```python
from build123d import *

# Parameters (mm, degrees)
SKETCH1_R           = 150
BOSS_EXTRUDE1_DEPTH = 3
SKETCH2_R           = 3.5
CUT_EXTRUDE1_DEPTH  = 3
CIRPATTERN1_COUNT   = 3
SKETCH3_R           = 2
CUT_EXTRUDE2_DEPTH  = 3
SKETCH4_R           = 15
CUT_EXTRUDE3_DEPTH  = 3
SKETCH6_R           = 1.5
CUT_EXTRUDE5_DEPTH  = 3


with BuildPart() as part:
    # Sketch1 → Boss-Extrude1 (new body)
    with BuildSketch(Plane.XY):
        Circle(SKETCH1_R)
    extrude(amount=BOSS_EXTRUDE1_DEPTH)

    # Sketch2 → Cut-Extrude1 (cut)
    with BuildSketch(Plane(origin=(0, 0, 0), x_dir=(-1, 0, 0), z_dir=(0, 0, -1))):
        with Locations((-84.532410842, 88.488821425)):
            Circle(SKETCH2_R)
        with Locations(Location((-112.064079787, 49.169523299, 0), (0, 0, 180))):
            Circle(SKETCH2_R)
    cut_extrude1 = extrude(amount=-CUT_EXTRUDE1_DEPTH, mode=Mode.SUBTRACT)

    # CirPattern1: Cut-Extrude1 ×3 about axis
    cirpattern1_axis = Axis((0, 0, 0), (0, 0, 1))
    for i in range(1, CIRPATTERN1_COUNT):
        add(cut_extrude1.rotate(cirpattern1_axis, i * 360 / CIRPATTERN1_COUNT), mode=Mode.SUBTRACT)

    # Sketch3 → Cut-Extrude2 (cut)
    with BuildSketch(Plane(origin=(0, 0, 0), x_dir=(-1, 0, 0), z_dir=(0, 0, -1))):
        with Locations((-109.9539568, -12.654144936)):
            Circle(SKETCH3_R)
        with Locations((-80.370678478, -76.095690029)):
            Circle(SKETCH3_R)
    extrude(amount=-CUT_EXTRUDE2_DEPTH, mode=Mode.SUBTRACT)

    # Sketch4 → Cut-Extrude3 (cut)
    with BuildSketch(Plane(origin=(0, 0, 0), x_dir=(-1, 0, 0), z_dir=(0, 0, -1))):
        Circle(SKETCH4_R)
    extrude(amount=-CUT_EXTRUDE3_DEPTH, mode=Mode.SUBTRACT)

    # Sketch6 → Cut-Extrude5 (cut)
    with BuildSketch(Plane(origin=(0, 0, 0), x_dir=(-1, 0, 0), z_dir=(0, 0, -1))):
        with Locations((66.962630167, -75.769427615)):
            Circle(SKETCH6_R)
        with Locations((86.113741245, -91.839117858)):
            Circle(SKETCH6_R)
        with Locations((105.397369535, -68.857784564)):
            Circle(SKETCH6_R)
        with Locations((86.246258457, -52.788094322)):
            Circle(SKETCH6_R)
    extrude(amount=-CUT_EXTRUDE5_DEPTH, mode=Mode.SUBTRACT)


solid = part.part
```
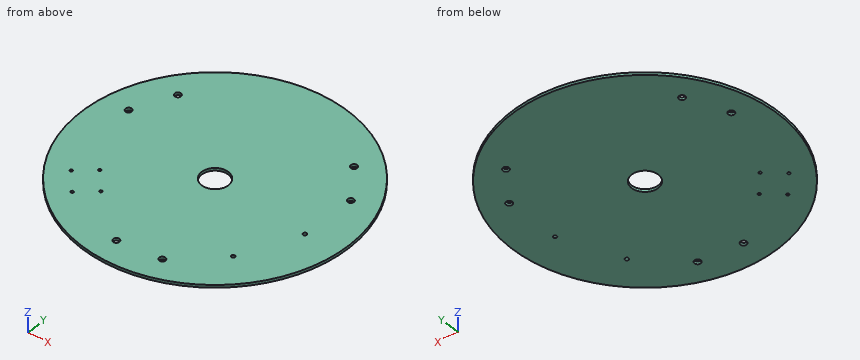
Part model, mm, in its own coordinate system. Round coordinates to 2 decimals unless told otherwise and drop trailing zeros. Loops run counter-clockwise (first coordinate to the right, second up) from the corner with the lowest first, then second, coordinate; pieces in that order, holes last.
1. Flat gauge pins, fed straight in: pin 1 (1 mm diameter, centred on x = -34, y = -31, fed in from -Z); pin 2 (1 mm diameter, centred on x = -39.5, z = 2.5, fed in from -Y); pin 3 (1.5 mm diameter, centred on x = -94.5, z = 0.5, fed in from +Y). Where does each tip first touch, or does it go through?
Solutions:
pin 1: stops at z = 0
pin 2: stops at y = -144.84
pin 3: stops at y = 117.09
2. Drill centre lines: line 1 along Y through (x, z) = (81.5, 1.5); line 2 along Y through (x, z) = (-96.5, 1.1); line 3 along Y through (x, z) = (3.5, 0.7). Where is each one in solid material? Low to high.
Solutions:
line 1: y = -125.93 to -77.75, -74.45 to 86.74, 90.24 to 125.93
line 2: y = -114.84 to 69.68, 75.25 to 114.84
line 3: y = -149.96 to -14.59, 14.59 to 149.96
3. Slice it at A-A (x = 0). Give the cut face in (y, z), and give its area (3 significant figures).
Solutions:
outline: (-150, 0) - (-15, 0) - (-15, 3) - (-150, 3) - close; (15, 0) - (150, 0) - (150, 3) - (15, 3) - close
area: 810 mm2
4. Slice it at C-C (z = 2.5). Count the separate pieces of the cut face and the enclosed holes in it, and give its area (3 significant figures).
Solutions:
separate pieces: 1
enclosed holes: 13
area: 69,700 mm2
5. Slice it at D-D (x = 125.5). Give the cut face in (y, z).
Solutions:
outline: (-82.16, 0) - (82.16, 0) - (82.16, 3) - (-82.16, 3) - close
